Autodesk Inventor part; units mm, degrees
ref_plane "conn_XY" through (0, 0, 0) normal (1, 0, 0) x (0, 0, -1)
ref_plane "conn_YZ" through (0, 0, 0) normal (0, 0, -1) x (0, 1, 0)
ref_plane "conn_ZX" through (0, 0, 0) normal (0, 1, 0) x (1, 0, 0)
sketch "Sketch_1" plane through (0, 0, 0) normal (1, 0, 0) x (0, 1, 0)
  line L0 (-3.2079, 5.5563) -> (-6.4158, 0)
  line L1 (-6.4158, 0) -> (-3.2079, -5.5563)
  line L2 (-3.2079, -5.5563) -> (3.2079, -5.5563)
  line L3 (3.2079, -5.5563) -> (6.4158, 0)
  line L4 (6.4158, 0) -> (3.2079, 5.5563)
  line L5 (3.2079, 5.5563) -> (-3.2079, 5.5563)
extrude "Extrusion1" add sketch "Sketch_1" along normal blind 3.9624
sketch "Fine_Thread" plane through (0, 0, 0) normal (0, 0, 1) x (1, 0, 0)
  line L0 (3.9624, 0) -> (0, 0)
  line L1 (0, 0) -> (0, 3.175)
  line L2 (0, 3.175) -> (0.4915, 2.6835)
  line L3 (0.4915, 2.6835) -> (3.4709, 2.6835)
  line L4 (3.4709, 2.6835) -> (3.9624, 3.175)
  line L5 (3.9624, 3.175) -> (3.9624, 0)
  line L6 (3.9624, 0) -> (0, 0)
revolve "Revolution1" cut sketch "Fine_Thread" angle 360 about axis through (3.9624, 0, 0) along (1, 0, 0)
thread "Thread1"
sketch "Sketch_3" plane through (0, 0, 0) normal (0, 0, 1) x (1, 0, 0)
  line L0 (25.4, 0) -> (-25.4, 0)
  line L1 (-0.508, 5.5563) -> (0, 5.5563)
  line L2 (0, 5.5563) -> (1.9812, 8.9878)
  line L3 (1.9812, 8.9878) -> (3.9624, 5.5563)
  line L4 (3.9624, 5.5563) -> (4.4704, 5.5563)
  line L5 (4.4704, 5.5563) -> (4.4704, 56.3563)
  line L6 (4.4704, 56.3563) -> (-0.508, 56.3563)
  line L7 (-0.508, 56.3563) -> (-0.508, 5.5563)
revolve "Revolution2" cut sketch "Sketch_3" angle 360 about axis through (25.4, 0, 0) along (1, 0, 0)
ref_plane "conn_XY" through (0, 0, 0) normal (1, 0, 0) x (0, 0, -1)
ref_plane "conn_YZ" through (0, 0, 0) normal (0, 0, -1) x (0, 1, 0)
ref_plane "conn_ZX" through (0, 0, 0) normal (0, 1, 0) x (1, 0, 0)
properties part number "PN1972-015_NUT1/4-28-UNF" material "Stainless Steel"
Work out the finished part from the listing and answer in its coordinate system (mm). Give positions to 0.01 mm unless a question says otherwise; leave off trailing zeros. Order: outer loops, then holes, each group sorted by start corner. A loop starts at its lowest first (then second) coordinate and runs counter-clockwise, first axis right, second up. Notation, with made-up numbers: (87, 24.5) -> (136, 24.5) arc R11 ccw to (136, 36.5) -> close; hole circle Ø3 at (8.5, 74.5). An arc over 180 degrees is marked (long way). One line per item, written item: value.
Item 1: Straight lines are drawn through the part: probe 1 along Z at (x, y) = (2.25, 0); probe 2 along Z at (x, y) = (2.1, -2); probe 3 along Y at (x, z) = (3.3, 2). For each, find the intervals that lie inside material, in ascending order.
Answer sheet:
probe 1: -5.56 to -2.68, 2.68 to 5.56
probe 2: -5.56 to -1.79, 1.79 to 5.56
probe 3: -5.26 to -1.79, 1.79 to 5.26
Item 2: A flat-ended cylindrical pin translates along its axis: P1, Ø1.5, axis at x = 3, z = 3.5, coming from the +Y side. Find the tip coordinate at first contact, or state that the pin passes through.
Answer sheet:
P1: y = 4.83
Item 3: Determine the mould class of faces 1 (the flat face through (3.962, 2.4, -2.4)), 2 (the conical face through (0.14, 2.9, 5.02)), 3 (the cylindrical face through (2, 2.56, 0.81)), 4 (the conical face through (3.823, -2.901, 5.019)) for opening direction Y: released by +Y, released by -Y, zero draft, split by the parting line, or undercut.
Answer sheet:
face 1: zero draft
face 2: released by +Y
face 3: undercut
face 4: released by -Y
Item 4: Find section A-A, the plane x = 2.75. Give the vertices of the cut face in (y, z).
Answer sheet:
outline: (-6.42, 0) -> (-3.21, -5.56) -> (3.21, -5.56) -> (6.42, 0) -> (3.21, 5.56) -> (-3.21, 5.56) -> close; hole circle Ø5.37 at (0, 0)
Item 5: Find section B-B, the plane x = 3.7. Give the vertices of the cut face in (y, z), plus the area to 3 significant figures.
Answer sheet:
outline: (-5.96, -0.79) -> (-3.67, -4.76) arc R6.01 ccw to (-2.29, -5.56) -> (2.29, -5.56) arc R6.01 ccw to (3.67, -4.76) -> (5.96, -0.79) arc R6.01 ccw to (5.96, 0.79) -> (3.67, 4.76) arc R6.01 ccw to (2.29, 5.56) -> (-2.29, 5.56) arc R6.01 ccw to (-3.67, 4.76) -> (-5.96, 0.79) arc R6.01 ccw to start; hole circle Ø5.83 at (0, 0)
area: 78.5 mm²
